For this review, use the dimensioned drawing (mm, ordinates from the lowest corner) and the shaded views. A direction names the side the tool comes from. Round coordinates to 2 decimals unless told otherwise and drop trailing zeros. Write each loop counter-clockwise with the first axis right and the second up, starting at its lowest first coordinate (ties: lowest second). Pieces come first, ordered by that corner, then holes. Notation, with made-up numbers: M 33,39.25 L 50,39.25 A9 cw 50,47.25 Z; hole C 18,80 d9. An arc over 180 degrees is marked long. Use CSV: the item, a comma, the result in double quotes.
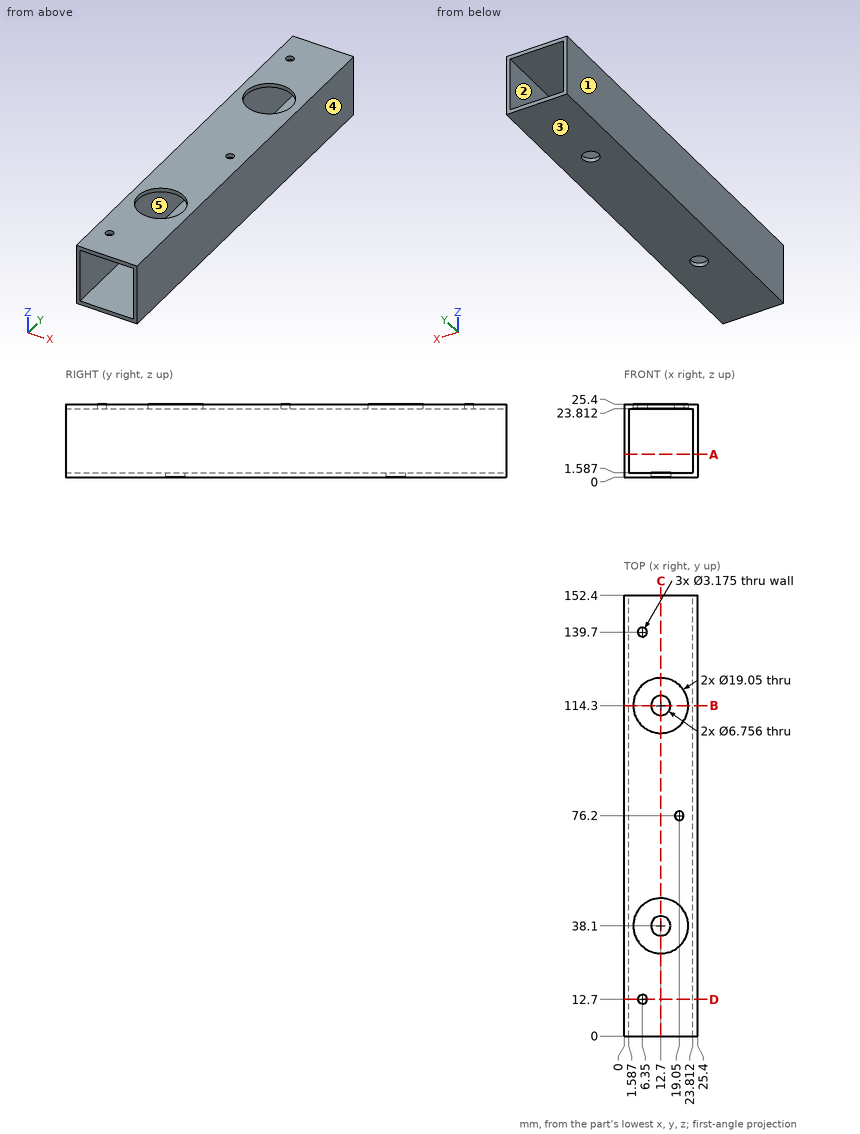
1) Add section C-C on x = 12.7. Write out the cut boundary in (y, z) (1 decimal).
Answers:
outline,"M 0,0 L 34.7,0 L 34.7,1.6 L 0,1.6 Z; M 0,23.8 L 28.6,23.8 L 28.6,25.4 L 0,25.4 Z; M 41.5,0 L 110.9,0 L 110.9,1.6 L 41.5,1.6 Z; M 47.6,23.8 L 104.8,23.8 L 104.8,25.4 L 47.6,25.4 Z; M 117.7,0 L 152.4,0 L 152.4,1.6 L 117.7,1.6 Z; M 123.8,23.8 L 152.4,23.8 L 152.4,25.4 L 123.8,25.4 Z"
2) The part is to be moulded in two halves that separate along X. For the marked faces 3, 4 and 5, say which applies: released by +X, released by -X, zero draft, split by the parting line, or undercut.
Answers:
face 3,"zero draft"
face 4,"released by +X"
face 5,"undercut"
3) Add section D-D on y = 12.7. Write out the cut boundary in (x, z), then the cut area to 3 significant figures.
Answers:
outline,"M 0,0 L 25.4,0 L 25.4,25.4 L 7.94,25.4 L 7.94,23.81 L 23.81,23.81 L 23.81,1.59 L 1.59,1.59 L 1.59,23.81 L 4.76,23.81 L 4.76,25.4 L 0,25.4 Z"
area,"146 mm²"
4) Wall thickness on line 1 along Y through (x, z) = (12.7, 25.15) (1 decimal); line 2 along X through (y, z) = (34, 7): over which ranges is each line inside the solid? List them lowest first. Write a range as [from, to].
Answers:
line 1,"[0, 28.6], [47.6, 104.8], [123.8, 152.4]"
line 2,"[0, 1.59], [23.81, 25.4]"
5) Machinability: for the marked faces 1 and 2, which of the approach directions +Z, -Z, +X, -X, +Y, -Y give a long, thin tool a straight path to every point of the face, cutting with its end or side? Answer none if there is none.
Answers:
face 1,"+Z, -Z, -X, +Y, -Y"
face 2,"+Y, -Y"
6) For pin 1 Ø6 at (x, z) = (4.5, 22.5) entering from -Y; pin 2 Ø4 at (x, z) = (13, 20) entering from +Y; pin 3 Ø3 at (x, y) = (19.05, 76.2) entering from +Z, all flat-tipped, find the tip position at first contact; note any pin that passes through.
Answers:
pin 1,"y = 0"
pin 2,"through"
pin 3,"z = 1.59"
7) Add section B-B on y = 114.3. Write out the cut boundary in (x, z) (1 decimal).
Answers:
outline,"M 0,0 L 9.3,0 L 9.3,1.6 L 1.6,1.6 L 1.6,23.8 L 3.2,23.8 L 3.2,25.4 L 0,25.4 Z; M 16.1,0 L 25.4,0 L 25.4,25.4 L 22.2,25.4 L 22.2,23.8 L 23.8,23.8 L 23.8,1.6 L 16.1,1.6 Z"
8) Add section A-A on z = 8. Write out the cut boundary in (x, y).
Answers:
outline,"M 0,0 L 1.59,0 L 1.59,152.4 L 0,152.4 Z; M 23.81,0 L 25.4,0 L 25.4,152.4 L 23.81,152.4 Z"
